Autodesk Fusion 360 part; units mm, degrees
sketch "Sketch1" plane through (0, 0, 0) normal (1, 0, 0) x (0, 1, 0)
  line L0 (0, 0) -> (20, 0)
  line L1 (20, 0) -> (20, 60)
  line L2 (20, 60) -> (0, 60)
  line L3 (0, 60) -> (0, 0)
  line L4 (5, 60) -> (5, 0)
  arc A0 (1, 0) -> (1, 60) centre (-448.5, 30) ccw
  arc A1 (3, 0) -> (3, 60) centre (-446.5, 30) ccw
  line L5 (0, 30) -> (5, 30) construction
  line L6 (2, 30) -> (2.3932, 29.5453) construction
  line L7 (4, 30) -> (3.7548, 30.2991) construction
  dimension "d3" = 60
  dimension "d4" = 20
  dimension "d5" = 5
  dimension "d6" = 1
  dimension "d7" = 2
  dimension "d8" = 1
  dimension "d9" = 2
  dimension "d16" = 2
  dimension "d17" = 2
extrude "Extrude2" add sketch "Sketch1" along normal blind 3
extrude "Extrude3" add sketch "Sketch1" against normal blind 15 contours L0 L2 L3 A0 | L0 L2 L4 A1
equation "d8 = d6"
equation "d9 = d7"
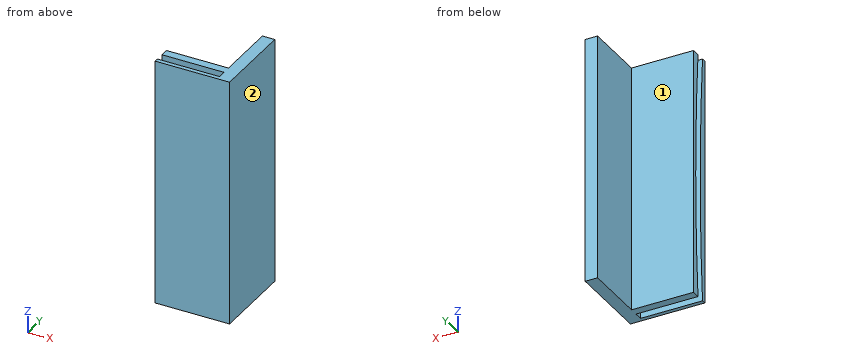
Source: CAD feature listing. Evaluate the final solid. Frame: model axes, mm. Face numbers are marked on the shaded views. A direction names the side the tool comes from. Coordinates: 2 decimals unless noted, no trailing zeros. Loops run counter-clockwise (first coordinate to the right, second up) from the corner with the lowest first, then second, coordinate; pieces in that order, holes last. Notation, with made-up numbers: (-34, 81) - (-3, 81) arc R37 cw to (-3, 117) - close; hole circle Ø7 at (49, 62). An arc over 180 degrees is marked (long way). Answer as CSV lines item,"result".
1. Section B-B (y = 8.5). Return loops of the section in (x, z), then the cut area to 3 significant figures.
Established:
outline,"(0, 0) - (3, 0) - (3, 60) - (0, 60) - close"
area,"180 mm2"
2. Section C-C (z = 23). Return loops of the section in (x, y).
Established:
outline,"(-15, 0) - (3, 0) - (3, 20) - (0, 20) - (0, 5) - (-15, 5) - (-15, 3.95) - (0, 3.95) - (0, 1.95) - (-15, 1.95) - close"
3. Contact query for flat-ended pins moving along their axis: pin 1 (5 mm diameter, centred on y = 12.5, z = 18.5, fed in from -X); pin 2 (4.5 mm diameter, centred on x = -7, z = 41.5, fed in from +Y). Output: stop coordinate, or through.
Established:
pin 1,"stops at x = 0"
pin 2,"stops at y = 5"
4. Reachability of the marked faces 1 and 2 from +Z, -Z, +X, -X, +Y, -Y: full face, straight path, thin tool, end or side. Return the list, or none.
Established:
face 1,"+Z, -Z, -X, +Y"
face 2,"+Z, -Z, +X, +Y, -Y"
5. Ray query, line 1 (Y direction, x = -13.5, z = 33); line 2 (X direction, y = 7.5, z = 45.5); line 3 (Y direction, x = -3.25, z = 4). Return the intervals inside material, ascending.
Established:
line 1,"y = 0 to 1.99, 3.99 to 5"
line 2,"x = 0 to 3"
line 3,"y = 0 to 1.25, 3.25 to 5"
6. Section A-A (x = -10). Return loops of the section in (y, z).
Established:
outline,"(0, 0) - (1, 0) arc R450.5 ccw to (1, 60) - (0, 60) - close; (3, 0) - (5, 0) - (5, 60) - (3, 60) arc R450.5 cw to start"
